```python
from build123d import *

# Parameters (mm, degrees)
SKETCH1_R               = 60.75
SKETCH1_R_2             = 45
BOSS_EXTRUDE1_DEPTH     = 4
SKETCH2_R               = 49
SKETCH2_R_2             = 45
BOSS_EXTRUDE2_DEPTH     = 52
SKETCH3_W               = 8
SKETCH3_H               = 38
SKETCH3_W_2             = 15
SKETCH3_H_2             = 8
BOSS_EXTRUDE3_DEPTH     = 13
SKETCH4_W               = 10
SKETCH4_H               = 23
CUT_EXTRUDE1_DEPTH      = 8
CUT_EXTRUDE2_REACH      = 111.593
CUT_EXTRUDE2_END_RADIUS = 49
SKETCH5_R               = 5
SKETCH6_R               = 1.4
CUT_EXTRUDE3_DEPTH      = 7.2
BOSS_EXTRUDE4_DEPTH     = 4
SKETCH8_R               = 2.5
CUT_EXTRUDE4_DEPTH      = 4


with BuildPart() as part:
    # Sketch1 → Boss-Extrude1 (new body)
    with BuildSketch(Plane(origin=(0, 0, 0), x_dir=(1, 0, 0), z_dir=(0, 1, 0))):
        with Locations(Location((0, 0, 0), (0, 0, 270))):
            Circle(SKETCH1_R)
        with Locations(Location((0, 0, 0), (0, 0, 270))):
            Circle(SKETCH1_R_2, mode=Mode.SUBTRACT)
    extrude(amount=BOSS_EXTRUDE1_DEPTH)

    # Sketch2 → Boss-Extrude2 (add)
    with BuildSketch(Plane(origin=(0, 4, 0), x_dir=(1, 0, 0), z_dir=(0, 1, 0))):
        with Locations(Location((0, 0, 0), (0, 0, 90))):
            Circle(SKETCH2_R)
        with Locations(Location((0, 0, 0), (0, 0, 270))):
            Circle(SKETCH2_R_2, mode=Mode.SUBTRACT)
    extrude(amount=BOSS_EXTRUDE2_DEPTH)

    # Sketch3 → Boss-Extrude3 (add, symmetric)
    with BuildSketch(Plane.XY):
        with Locations((15.25, 19)):
            Rectangle(SKETCH3_W, SKETCH3_H)
        with Locations((-39.25, 34)):
            Rectangle(SKETCH3_W_2, SKETCH3_H_2)
    extrude(amount=BOSS_EXTRUDE3_DEPTH, both=True)


with BuildPart() as boss_extrude3_piece_1:
    # of the separate pieces the step leaves, piece 1, a body of its own (boss_extrude3_pieces)
    add(part.part.solids().sort_by_distance((0, 0, 60.75))[0])

    # Cut-Extrude2: up to this cylinder (the profile starts inside it)
    cut_extrude2_end = Plane(origin=(0, 19, 0), z_dir=(0, -1, 0)) * Cylinder(CUT_EXTRUDE2_END_RADIUS, 322.186, mode=Mode.PRIVATE)
    # Sketch5 → Cut-Extrude2 (cut, up to the surface)
    with BuildSketch(Plane.ZY.offset(-11.25), mode=Mode.PRIVATE) as cut_extrude2_sk1:
        with Locations(Location((0, 19, 0), (0, 0, 270))):
            Circle(SKETCH5_R)
    cut_extrude2_tool1 = extrude(cut_extrude2_sk1.sketch, amount=-CUT_EXTRUDE2_REACH, mode=Mode.PRIVATE) & cut_extrude2_end
    add(cut_extrude2_tool1.solids().sort_by_distance((11.25, 19, 0))[0], mode=Mode.SUBTRACT)


with BuildPart() as boss_extrude3_piece_2:
    # of the separate pieces the step leaves, piece 2, a body of its own (boss_extrude3_pieces)
    add(part.part.solids().sort_by_distance((11.25, 0, -13))[0])

    # Sketch4 → Cut-Extrude1 (cut)
    with BuildSketch(Plane.ZY.offset(-11.25)):
        with Locations((0, 16.5)):
            Rectangle(SKETCH4_W, SKETCH4_H)
    extrude(amount=-CUT_EXTRUDE1_DEPTH, mode=Mode.SUBTRACT)


with BuildPart() as cut_extrude3_tool:
    # Sketch6 → Cut-Extrude3 (new body)
    with BuildSketch(Plane(origin=(0, 38, 0), x_dir=(1, 0, 0), z_dir=(0, 1, 0))):
        with Locations(Location((-34.25, -5, 0), (0, 0, 270))):
            Circle(SKETCH6_R)
        with Locations(Location((13.75, -5, 0), (0, 0, 270))):
            Circle(SKETCH6_R)
        with Locations(Location((13.75, 5, 0), (0, 0, 90))):
            Circle(SKETCH6_R)
        with Locations(Location((-34.25, 5, 0), (0, 0, 90))):
            Circle(SKETCH6_R)
    extrude(amount=-CUT_EXTRUDE3_DEPTH)


with BuildPart() as boss_extrude3_piece_1_1:
    add(boss_extrude3_piece_1.part)

    # Cut-Extrude3: cut by cut_extrude3_tool
    add(cut_extrude3_tool.part, mode=Mode.SUBTRACT)



with BuildPart() as boss_extrude3_piece_2_1:
    add(boss_extrude3_piece_2.part)

    # Cut-Extrude3: cut by cut_extrude3_tool
    add(cut_extrude3_tool.part, mode=Mode.SUBTRACT)


with BuildPart() as boss_extrude3_piece_1_2:
    add(boss_extrude3_piece_1_1.part)

    add(boss_extrude3_piece_2_1.part)  # Boss-Extrude4 merges Boss-Extrude3 piece 2
    # Sketch7 → Boss-Extrude4 (add)
    with BuildSketch(Plane.XZ):
        with BuildLine():
            Line((11.25, -13), (25.249838503, -37.248431585))
            ThreePointArc((25.249838503, -37.248431585), (45, 0), (25.249838503, 37.248431585))
            Line((25.249838503, 37.248431585), (11.25, 13))
            Line((11.25, 13), (11.25, -13))
        make_face()
        with BuildLine():
            Line((24.25, 19.516660498), (27.361802413, 24.906460381))
            ThreePointArc((27.361802413, 24.906460381), (37, 0), (27.361802413, -24.906460381))
            Line((27.361802413, -24.906460381), (24.25, -19.516660498))
            Line((24.25, -19.516660498), (24.25, 19.516660498))
        make_face(mode=Mode.SUBTRACT)
    extrude(amount=-BOSS_EXTRUDE4_DEPTH)

    # Sketch8 → Cut-Extrude4 (cut)
    with BuildSketch(Plane(origin=(0, 4, 0), x_dir=(1, 0, 0), z_dir=(0, 1, 0))):
        with Locations(Location((-55, 0, 0), (0, 0, 270))):
            Circle(SKETCH8_R)
        with Locations(Location((0, 55, 0), (0, 0, 270))):
            Circle(SKETCH8_R)
        with Locations(Location((55, 0, 0), (0, 0, 270))):
            Circle(SKETCH8_R)
        with Locations(Location((0, -55, 0), (0, 0, 270))):
            Circle(SKETCH8_R)
    extrude(amount=-CUT_EXTRUDE4_DEPTH, mode=Mode.SUBTRACT)


solid = boss_extrude3_piece_1_2.part
```
Check sheet for the modelled part. Datum: model origin and axes. Units: mm. A direction names the side the tool comes from. Round coordinates to 2 decimals unless told otherwise and drop trailing zeros. Order: outer loops, then holes, each group sorted by start corner. A loop starts at its lowest first (then second) coordinate and runs counter-clockwise, first axis right, second up. Notation, with made-up numbers: (29, -8.75) - (79, -8.75) arc R12 cw to (79, -0.75) - close; hole circle Ø9 at (-27.5, 73). An arc over 180 degrees is marked (long way). Answer as CSV lines item,"result". Start each with the question number.
1) Section check A-A (y = 34). Record the cut outline in (x, z), then the cut area to 3 significant figures.
2) Section check C-C (x = 0). Record the cut outline in (y, z).
3) Depth check by flat-ended pin: pin 1 (3 mm diameter, centred on x = -34.5, z = 5.5, fed in from +Y); pin 2 (11.5 mm diameter, centred on y = 19, z = 0, fed in from +X); pin 3 (2.5 mm diameter, centred on x = -38, y = 34, fed in from -Z); pin 4 (4.5 mm diameter, centred on x = 0, z = -55, fed in from -Y). Enter the tip coordinate at first touch or a pass-through.
4) Tool access check on faces 1 (the face through (13, 0, 1)), 2 (the face through (25.8, 2, 22.2)), 3 (the face through (15, 38, 0)), 4 (the face through (15, 5, 0)), 5 (the face through (22, 56, -40)). Record the directions out of +Z, -Z, +X, -X, +Y, -Y that give a thin tool (end or side, any length) a straight path to the whole face; none if there is none.
5) Draft check along Y on faces 6 (the face through (-38, 30, 0)), 7 (the face through (15, 21, -13)), 8 (the face through (15, 16, 5)). Enter one of: +Y half, -Y half, draft (parallel to the pull), parting line (faces both ways), or undercut.
6) Section check B-B (y = 8.5). Record the cut outline in (x, z).
7) Scan lines: probe 1 along X at (y, z) = (27.5, 1.5) (3 decimals); probe 2 along Z at (x, y) = (-34, 34); probe 3 along Y at (x, z) = (47.7, 0). Record each from-to range of solid material in increasing order.
8) Section check D-D (x = -55). Record the cut outline in (y, z), then the cut area to 3 significant figures.
Determined:
1,outline,"circle Ø98 at (0, 0); (11.25, -13) - (19.25, -13) - (19.25, 13) - (11.25, 13) - close; hole (-43.08, -13) arc R45 ccw (long way) to (-43.08, 13) - (-31.75, 13) - (-31.75, -13) - close; hole circle Ø2.8 at (-34.25, -5); hole circle Ø2.8 at (-34.25, 5); hole circle Ø2.8 at (13.75, -5); hole circle Ø2.8 at (13.75, 5)"
1,area,"1,690 mm^2"
2,outline,"(0, -60.75) - (4, -60.75) - (4, -57.5) - (0, -57.5) - close; (0, -52.5) - (4, -52.5) - (4, -49) - (56, -49) - (56, -45) - (0, -45) - close; (0, 45) - (56, 45) - (56, 49) - (4, 49) - (4, 52.5) - (0, 52.5) - close; (0, 57.5) - (4, 57.5) - (4, 60.75) - (0, 60.75) - close"
3,pin 1,"y = 38"
3,pin 2,"x = 49"
3,pin 3,"z = -32.41"
3,pin 4,"through"
4,face 1,"+Z, -Z, +X, -X, -Y"
4,face 2,"+Y, -Y"
4,face 3,"+Y"
4,face 4,"none"
4,face 5,"+Z, -Z, +X, -X, +Y"
5,face 6,"-Y half"
5,face 7,"draft"
5,face 8,"undercut"
6,outline,"circle Ø98 at (0, 0); (11.25, -13) - (19.25, -13) - (19.25, -5) - (11.25, -5) - close; (11.25, 5) - (19.25, 5) - (19.25, 13) - (11.25, 13) - close; hole circle Ø90 at (0, 0)"
7,probe 1,"-48.977 to -44.975, 44.975 to 48.977"
7,probe 2,"-35.28 to -29.48, -13 to -6.38, -3.62 to 3.62, 6.38 to 13, 29.48 to 35.28"
7,probe 3,"0 to 14, 24 to 56"
8,outline,"(0, -25.8) - (4, -25.8) - (4, -2.5) - (0, -2.5) - close; (0, 2.5) - (4, 2.5) - (4, 25.8) - (0, 25.8) - close"
8,area,"186 mm^2"
